Here's the drawing with two shaded views (mm, measured from the low corner). I have some questions. Round coordinates to 2 decimals unless told otherwise and drop trailing zeros. Order: outer loops, then holes, each group sorted by start corner. A loop starts at its lowest first (then second) coordinate and runs counter-clockwise, first axis right, second up.
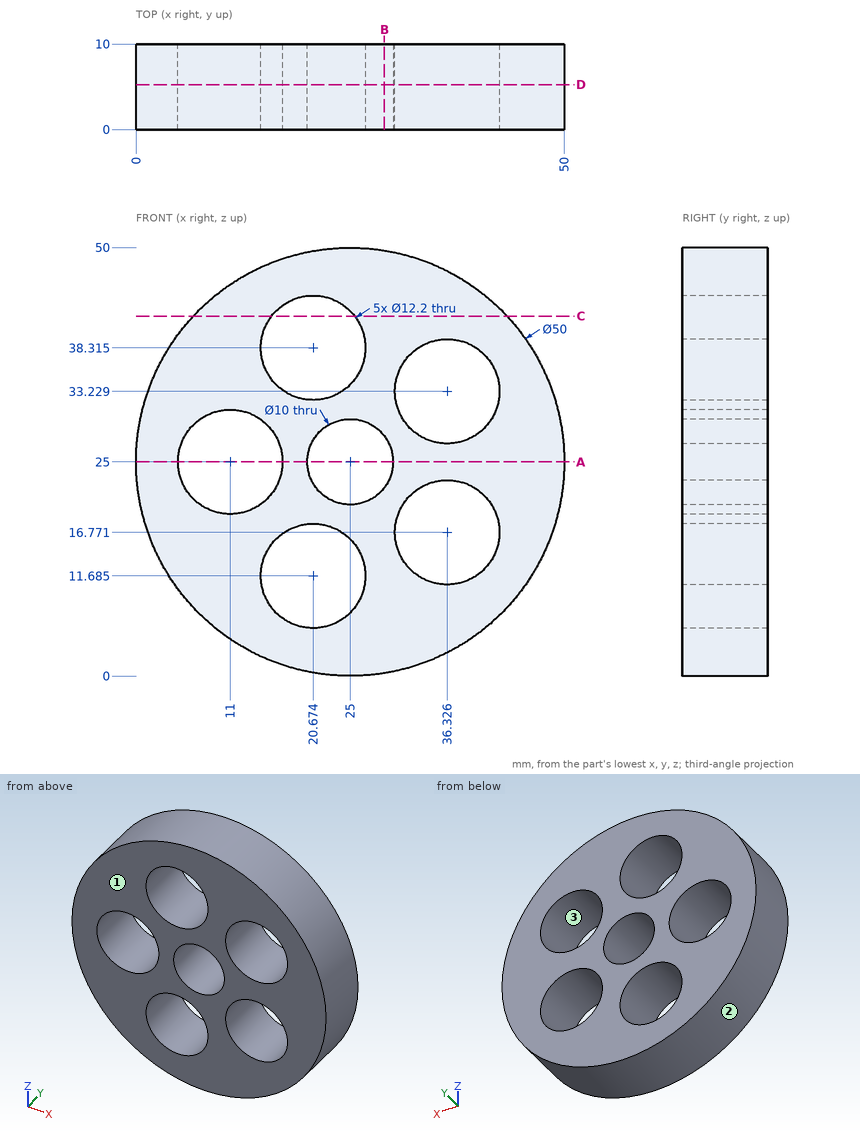
1. If we section it at D-D, the plane y = 5.25: Write out the boundary of the cut face in (x, z) (1 decimal), and give its area (3 significant figures).
Evaluation:
outline: circle Ø50 at (25, 25); hole circle Ø12.2 at (11, 25); hole circle Ø12.2 at (20.7, 11.7); hole circle Ø12.2 at (20.7, 38.3); hole circle Ø10 at (25, 25); hole circle Ø12.2 at (36.3, 16.8); hole circle Ø12.2 at (36.3, 33.2)
area: 1,300 mm2
2. I'm going to push flat-ended pins straight in: P1, Ø1, axis at y = 5, z = 27, coming from the +X side (3 decimals); P2, Ø1, axis at x = 14, y = 6, coming from the +Z side; P3, Ø1.5, axis at x = 6, y = 3.5, coming from the -Z side. Where does each tip first touch, or does it pass through?
Evaluation:
P1: stops at x = 49.955
P2: stops at z = 47.69
P3: stops at z = 7.91
3. If we section it at B-B, the plane x = 29: Write out the boundary of the cut face in (y, z).
Evaluation:
outline: (0, 0.32) - (10, 0.32) - (10, 22) - (0, 22) - close; (0, 28) - (10, 28) - (10, 49.68) - (0, 49.68) - close
4. If we section it at A-A, the plane z = 25: Write out the boundary of the cut face in (x, y), and give its area (3 significant figures).
Evaluation:
outline: (0, 0) - (4.9, 0) - (4.9, 10) - (0, 10) - close; (17.1, 0) - (20, 0) - (20, 10) - (17.1, 10) - close; (30, 0) - (50, 0) - (50, 10) - (30, 10) - close
area: 278 mm2
5. If we mould it in two halves opening along Z, with no side actions, what happens to the marked faces 1, 2 and 3? For each: released by +Z, released by -Z, zero draft, split by the parting line, or undercut.
Evaluation:
face 1: zero draft
face 2: split by the parting line
face 3: undercut
6. I need wall thicknesses on probe 1 along Z at (x, y) = (32.5, 9); probe 2 along Z at (x, y) = (22.5, 3.75) (1 decimal); probe 3 along Z at (x, y) = (25, 6.5) (1 decimal). Which ranges of each line are inside material? Lowest first, please.
Evaluation:
probe 1: z = 1.15 to 12.02, 21.52 to 28.48, 37.98 to 48.85
probe 2: z = 0.1 to 5.9, 17.5 to 20.7, 29.3 to 32.5, 44.1 to 49.9
probe 3: z = 0 to 7.4, 16 to 20, 30 to 34, 42.6 to 50
7. If we section it at C-C, the plane z = 42: Write out the boundary of the cut face in (x, y) (1 decimal), and give its area (3 significant figures).
Evaluation:
outline: (6.7, 0) - (15.8, 0) - (15.8, 10) - (6.7, 10) - close; (25.5, 0) - (43.3, 0) - (43.3, 10) - (25.5, 10) - close
area: 269 mm2
